```python
from build123d import *

# Parameters (mm, degrees)
SKETCH_R      = 5
PAD_DEPTH     = 3
SKETCH001_R   = 6.5
SKETCH001_R_2 = 5
PAD001_DEPTH  = 3.5


with BuildPart() as part:
    # Sketch → Pad (new body)
    with BuildSketch(Plane.XY):
        Polygon((7.505553, 0), (3.752777, 6.5), (-3.752777, 6.5), (-7.505553, 0), (-3.752777, -6.5), (3.752777, -6.5), align=None)
        Circle(SKETCH_R, mode=Mode.SUBTRACT)
    extrude(amount=PAD_DEPTH)

    # Sketch001 (on Face9 of Pad) → Pad001 (join)
    with BuildSketch(Plane.XY.offset(3)):
        Circle(SKETCH001_R)
        Circle(SKETCH001_R_2, mode=Mode.SUBTRACT)
    extrude(amount=PAD001_DEPTH)


solid = part.part
```
Verification items for the finished model (mm, model axes). A direction names the side the tool comes from. Give positions to 0.01 mm unless a question says otherwise; leave off trailing zeros. Order: outer loops, then holes, each group sorted by start corner. A loop starts at its lowest first (then second) coordinate and runs counter-clockwise, first axis right, second up. Notation, with made-up numbers: (-33, 33) - (26, 33) arc R17 ccw to (26, 47) - close; hole circle Ø1 at (-39, -39.75). An arc over 180 degrees is marked (long way). Answer as CSV lines item,"result". Start each with the question number.
Item 1: Material ranges on L1, parallel to Y at x = 0, z = 5; L2, parallel to X at y = 4.5, z = 5.5; L3, parallel to X at y = -3.5, z = 1, recorded low to high.
Item 2: Section check B-B, the plane y = -4.75. Record the boundary of the cut face in (x, z), plus the area to 3 significant figures.
Item 3: Access from +Z, -Z, +X, -X, +Y, -Y to the whole of each face (thin tool, end or side, straight path). Record for faces 1 (the face through (3, 6, 3)), 2 (the face through (-3, 6, 3)), 3 (the face through (-3, -6, 3)), 4 (the face through (-5.158, -3.955, 4.726)), 5 (the face through (3, -6, 3)).
Item 4: Mould release check, pull along X, two halves, no side actions. Record for faces 6 (the face through (0, -6.5, 1)), 7 (the face through (-1.08, -4.88, 3.2)), 8 (the face through (5.6, -3.3, 1.5)): released by +X, released by -X, zero draft, split by the parting line, or undercut.
Item 5: Section check D-D, the plane x = 5.25. Record the boundary of the cut face in (y, z), plus the area to 3 significant figures.
Item 6: Section check C-C, the plane x = -1.25. Record the boundary of the cut face in (y, z), plus the area to 3 significant figures.
Item 7: Gauge pin test, flat ends, axial feed: pin 1 (1.5 mm diameter, centred on y = 5, z = 3, fed in from -X); pin 2 (6 mm diameter, centred on x = 0, y = 0, fed in from +Z); pin 3 (1.5 mm diameter, centred on y = -0.5, z = 5, fed in from +X). Record the tip position at first contact, or that the pin passes through.
Item 8: Section check A-A, the plane z = 2.25. Record the boundary of the cut face in (x, y), plus the area to 3 significant figures.
Filled in:
1,L1,"-6.5 to -5, 5 to 6.5"
1,L2,"-4.69 to -2.18, 2.18 to 4.69"
1,L3,"-5.48 to -3.57, 3.57 to 5.48"
2,outline,"(-4.76, 0) - (-1.56, 0) - (-1.56, 6.5) - (-4.44, 6.5) - (-4.44, 3) - (-4.76, 3) - close; (1.56, 0) - (4.76, 0) - (4.76, 3) - (4.44, 3) - (4.44, 6.5) - (1.56, 6.5) - close"
2,area,"39.3 mm^2"
3,face 1,"+Z, +X, +Y"
3,face 2,"+Z, -X, +Y"
3,face 3,"+Z, -X, -Y"
3,face 4,"+Z"
3,face 5,"+Z, +X, -Y"
4,face 6,"zero draft"
4,face 7,"undercut"
4,face 8,"released by +X"
5,outline,"(-3.91, 0) - (3.91, 0) - (3.91, 3) - (3.83, 3) - (3.83, 6.5) - (-3.83, 6.5) - (-3.83, 3) - (-3.91, 3) - close"
5,area,"50.3 mm^2"
6,outline,"(-6.5, 0) - (-4.84, 0) - (-4.84, 6.5) - (-6.38, 6.5) - (-6.38, 3) - (-6.5, 3) - close; (4.84, 0) - (6.5, 0) - (6.5, 3) - (6.38, 3) - (6.38, 6.5) - (4.84, 6.5) - close"
6,area,"20.7 mm^2"
7,pin 1,"x = -5.05"
7,pin 2,"through"
7,pin 3,"x = 6.5"
8,outline,"(-7.51, 0) - (-3.75, -6.5) - (3.75, -6.5) - (7.51, 0) - (3.75, 6.5) - (-3.75, 6.5) - close; hole circle Ø10 at (0, 0)"
8,area,"67.8 mm^2"
